```python
from build123d import *

# Parameters (mm, degrees)
SKETCH_1_R               = 1.5
EXTRUDE_1_DEPTH          = 2
SKETCH_2_W               = 18
SKETCH_2_H               = 3
EXTRUDE_2_DEPTH          = 2.5
EXTRUDE_3_DEPTH          = 2.5
FILLET_1_R               = 0.5
FILLET_2_R               = 0.5
CUT_EXTRUDE_1_DEPTH      = 22.236760582
CUT_EXTRUDE_1_DEPTH_BACK = 10
SKETCH_6_R               = 1.35


with BuildPart() as part:
    # Sketch 1 → Extrude 1 (new body)
    with BuildSketch(Plane.XY):
        with BuildLine():
            Line((-6, 0), (-6, -8))
            Line((-6, -8), (-9, -8))
            Line((-9, -8), (-9, -11))
            Line((-9, -11), (9, -11))
            Line((9, -11), (9, -8))
            Line((9, -8), (6, -8))
            Line((6, -8), (6, 0))
            ThreePointArc((6, 0), (0, 6), (-6, 0))
        make_face()
        Circle(SKETCH_1_R, mode=Mode.SUBTRACT)
    extrude(amount=EXTRUDE_1_DEPTH)

    # Sketch 2 → Extrude 2 (add)
    with BuildSketch(Plane.XY.offset(2)):
        with Locations((0, -9.5)):
            Rectangle(SKETCH_2_W, SKETCH_2_H)
    extrude(amount=EXTRUDE_2_DEPTH)

    # Sketch 5 → Extrude 3 (add)
    with BuildSketch(Plane.XY.offset(2)):
        with BuildLine():
            Line((6, -1.75), (6, -8))
            Line((6, -8), (-6, -8))
            Line((-6, -8), (-6, -1.75))
            ThreePointArc((-6, -1.75), (0, -6.25), (6, -1.75))
        make_face()
    extrude(amount=EXTRUDE_3_DEPTH)

    # Fillet 1
    fillet_1_edges = [part.edges().sort_by_distance(p)[0] for p in [
        (-6, -1.75, 3.25),
    ]]
    fillet(fillet_1_edges, radius=FILLET_1_R)

    # Fillet 2
    fillet_2_edges = [part.edges().sort_by_distance(p)[0] for p in [
        (6, -1.75, 3.25),
    ]]
    fillet(fillet_2_edges, radius=FILLET_2_R)

    # Mirror 3: part across plane


with BuildPart() as part_1:
    add(part.part)
    add(part.part.mirror(Plane(origin=(0, 0, 4.5), x_dir=(1, 0, 0), z_dir=(0, 0, -1))))

    # Sketch 6 → Cut-Extrude 1 (cut, two sides: drawn at the far end of the back side and taken through both)
    with BuildSketch(Plane.XZ.offset(11).offset(-CUT_EXTRUDE_1_DEPTH_BACK)):
        with Locations(Location((0, 4.5, 0), (0, 0, 90))):
            Circle(SKETCH_6_R)
    extrude(amount=CUT_EXTRUDE_1_DEPTH + CUT_EXTRUDE_1_DEPTH_BACK, mode=Mode.SUBTRACT)


solid = part_1.part
```
For this review, take the finished solid that the model builds, in its own axes (mm). A direction names the side the tool comes from. Round coordinates to 2 decimals unless told otherwise and drop trailing zeros. Order: outer loops, then holes, each group sorted by start corner. A loop starts at its lowest first (then second) coordinate and runs counter-clockwise, first axis right, second up.
Q1. Machinability: for faces 4 (the flat face through (7, -8, 5)), 5 (the cylindrical face through (-1.5, 0.07, 8.01)), 6 (the cylindrical face through (5.66, -3.44, 4.46)), which of the approach directions +Z, -Z, +X, -X, +Y, -Y give a long, thin tool a straight path to every point of the face, cutting with its end or side? Answer none if there is none.
Findings below:
face 4: +Z, -Z, +X, +Y
face 5: +Z, -Z
face 6: +Y
Q2. We need section A-A, the plane z = 4.5. Give the boundary of the cut face in (x, y), plus the area to 3 significant figures.
Findings below:
outline: (-9, -11) - (-1.35, -11) - (-1.35, -6.1) arc R6.25 cw to (-5.09, -3.62) arc R0.5 ccw to (-6, -3.91) - (-6, -8) - (-9, -8) - close; (1.35, -11) - (9, -11) - (9, -8) - (6, -8) - (6, -3.91) arc R0.5 ccw to (5.09, -3.62) arc R6.25 cw to (1.35, -6.1) - close
area: 75.0 mm2
Q3. We need section D-D, the plane y = -7.5. Give the boundary of the cut face in (x, z), plus the area to 3 significant figures.
Findings below:
outline: (-6, 0) - (6, 0) - (6, 9) - (-6, 9) - close; hole circle Ø2.7 at (0, 4.5)
area: 102 mm2
Q4. Insertion check: P1, Ø2, axis at y = -1.5, z = 2, coming from the -X side; P2, Ø4, axis at x = -4, z = 1.5, coming from the +Y side; P3, Ø3.5, axis at x = -8, z = 4, coming from the +Y side. Each pin has a flat end and moves straight along its axis. Give the tip position at first contact, or say it passes through.
Findings below:
P1: stops at x = -6
P2: stops at y = 5.66
P3: stops at y = -8
Q5. Wall thickness on line 1 (Z direction, x = 1.25, y = -3.25); line 2 (Y direction, x = 0, z = 0.65); line 3 (X direction, y = -7.1, z = 4.5): over which ranges is each line inside the solid? List them lowest first.
Findings below:
line 1: z = 0 to 2, 7 to 9
line 2: y = -11 to -1.5, 1.5 to 6
line 3: x = -6 to -1.35, 1.35 to 6
Q6. We need section B-B, the plane y = -1.75. Give the boundary of the cut face in (x, z).
Findings below:
outline: (-6, 0) - (6, 0) - (6, 2) - (-6, 2) - close; (-6, 7) - (6, 7) - (6, 9) - (-6, 9) - close
Q7. We need section C-C, the plane z = 0.75. Give the boundary of the cut face in (x, y), plus the area to 3 significant figures.
Findings below:
outline: (-9, -11) - (9, -11) - (9, -8) - (6, -8) - (6, 0) arc R6 ccw to (-6, 0) - (-6, -8) - (-9, -8) - close; hole circle Ø3 at (0, 0)
area: 199 mm2
Q8. Mouldability with a two-part tool opening along X and no side actions: class faces 1 (the cylindrical face through (0, 6, 1)), 2 (the flat face through (-6, -5, 5)), 3 (the cylindrical face through (-5.66, -3.44, 4.46)) as pulls with the +X half, pulls with the -X half, needs draft (parallel to the pull), parting line crosses it, or undercut.
Findings below:
face 1: parting line crosses it
face 2: pulls with the -X half
face 3: undercut
